Model file for the job. Use its own axes, mm. Coordinates: 2 decimals unless noted, no trailing zeros. Loops run counter-clockwise (first coordinate to the right, second up) from the corner with the lowest first, then second, coordinate; pieces in that order, holes last. Notation, with made-up numbers: M 74.25,65.5 L 119.25,65.5 A30 cw 119.25,102.5 Z; hole C 53.5,-20.5 d10. An arc over 180 degrees is marked long. Write item = value, one per line. Start each with the question number.
Autodesk Fusion 360 part; units mm, degrees
sketch "Sketch1" plane through (0, 0, 0) normal (0, 0, 1) x (1, 0, 0)
  line L0 (-50, 100) -> (50, 100)
  line L1 (50, 100) -> (100, 50)
  line L2 (100, 50) -> (100, 0)
  line L3 (100, 0) -> (50, -50)
  line L4 (50, -50) -> (-50, -50)
  line L5 (-50, -50) -> (-100, 0)
  line L6 (-100, 0) -> (-100, 50)
  line L7 (-100, 50) -> (-50, 100)
extrude "Extrude1" add sketch "Sketch1" along normal blind 50
hole "Hole1" at (-1.9643, 26.0412, 50) direction (0, 0, -1) diameter 100 depth 60 tip angle 118
hole "Hole2" at (76.0323, 27.1251, 50) direction (0, 0, -1) diameter 20 depth 60 tip angle 118
hole "Hole3" at (-75.8603, 25.7082, 50) direction (0, 0, -1) diameter 20 depth 60 tip angle 118
Item 1: Cut at B-B (y = 73.5). Give the cut face in (x, z), plus the area to 3 significant figures.
Item 2: Cut at A-A (x = -69). Give the cut face in (y, z).
Item 3: Probe L1, parallel to Y at x = 70, z = 48; L2, parallel to Y at x = 14, z = 10; L3, parallel to X at y = 66, z = 8. List the from-to ranges inside material, lowest first.
Item 4: Cut at C-C (z = 32.5). Give the cut face in (x, y).
Item 5: Pin check, flat tips, straight feed: pin 1 Ø1 at (y, z) = (80.5, 38.5) entering from -X; pin 2 Ø4 at (y, z) = (81.5, 35.5) entering from +X; pin 3 Ø8 at (y, z) = (52.5, 18.5) entering from -X. Stop position of each tip, or through.
Item 6: Pull direction X, two halves, no side cores. Call faces 1 (the cylindrical face through (84.9, 22.5, 24.6)), 2 (the flat face through (75, -25, 25)), 3 (the flat face through (21, 76, 0)): +X half, -X half, draft (parallel to the pull), parting line (faces both ways), or undercut.
Item 7: Cut at D-D (x = 59.5). Give the cut face in (y, z).
Reported:
q1.outline = M -76.5,0 L -17.7,0 L -17.7,50 L -76.5,50 Z; M 13.77,0 L 76.5,0 L 76.5,50 L 13.77,50 Z
q1.area = 6,080 mm^2
q2.outline = M -31,0 L 18.43,0 L 18.43,50 L -31,50 Z; M 32.98,0 L 81,0 L 81,50 L 32.98,50 Z
q3.L1 = -30 to 19.15, 35.1 to 80
q3.L2 = -50 to -21.34, 73.42 to 100
q3.L3 = -84 to -32.02, 28.09 to 84
q4.outline = M -100,0 L -50,-50 L 50,-50 L 100,0 L 100,50 L 50,100 L -50,100 L -100,50 Z; hole C -75.86,25.71 d20; hole C -1.96,26.04 d100; hole C 76.03,27.13 d20
q5.pin_1 = -70
q5.pin_2 = 70.5
q5.pin_3 = -100
q6.face_1 = undercut
q6.face_2 = +X half
q6.face_3 = draft
q7.outline = M -40.5,0 L 90.5,0 L 90.5,50 L -40.5,50 Z
